Autodesk Inventor part; units mm, degrees
ref_plane "YZ Plane" through (0, 0, 0) normal (1, 0, 0) x (0, 1, 0)
ref_plane "XZ Plane" through (0, 0, 0) normal (0, 1, 0) x (-1, 0, 0)
ref_plane "XY Plane" through (0, 0, 0) normal (0, 0, 1) x (1, 0, 0)
sketch "Эскиз1" plane through (0, 0, 0) normal (0, 0, 1) x (1, 0, 0)
  line L0 (-69.2132, 0) -> (64.0355, 0)
  line L1 (0, -42.2487) -> (0, 42.2487)
  line L2 (-20, 25) -> (45, 25)
  line L3 (45, 25) -> (45, -25)
  line L4 (45, -25) -> (-20, -25)
  line L5 (-45, 0) -> (-45, 0)
  arc A0 (-20, 25) -> (-45, 0) centre (-20, 0) ccw
  arc A1 (-45, 0) -> (-20, -25) centre (-20, 0) ccw
  point P0 (0, 0)
  point P1 (-45, 25)
  dimension "d0" = 50
  dimension "d1" = 90
  dimension "d2" = 25
extrude "Выдавливание1" add sketch "Эскиз1" along normal blind 15
sketch "Эскиз2" plane through (0, 0, 15) normal (0, 0, 1) x (1, 0, 0)
  line L0 (45, -25) -> (45, 25)
  circle A0 centre (-10, 0) radius 14
  point P0 (0, 0)
  point P1 (30, 14.0013)
  point P2 (31.2898, -16.1928)
  dimension "d6" = 15
  dimension "d7" = 40
  dimension "d8" = 28
extrude "Выдавливание2" add sketch "Эскиз2" along normal blind 25
sketch "Эскиз3" plane through (-10, 0, 40) normal (0, 0, 1) x (1, 0, 0)
  point P0 (10, 0)
sketch "Эскиз4" plane through (-10, 0, 40) normal (0, 0, 1) x (1, 0, 0)
  point P0 (10, 0)
  point P1 (0, 0)
hole "Отверстие1" at (-10, 0, 40) direction (0, 0, -1) diameter 15.835 depth 30
chamfer "Фаска1" distance 2 angle 45 1 edges at (-10, 7.9175, 40)
sketch "Эскиз5" plane through (0, 0, 15) normal (0, 0, 1) x (1, 0, 0)
  line L0 (45, -25) -> (45, 25)
  circle A0 centre (-10, 0) radius 7.9175
  line L1 (-63, 0) -> (63, 0)
  line L2 (0, -35) -> (0, 35)
  point P0 (0, 0)
  point P1 (30, 15)
  point P2 (30, -15)
  dimension "d21" = 15
  dimension "d22" = 40
  dimension "d23" = 30
hole "Отверстие2" at (30, 15, 15) at (30, -15, 15) direction (0, 0, -1) diameter 10 end through all
properties part number "Основание дз курганова"
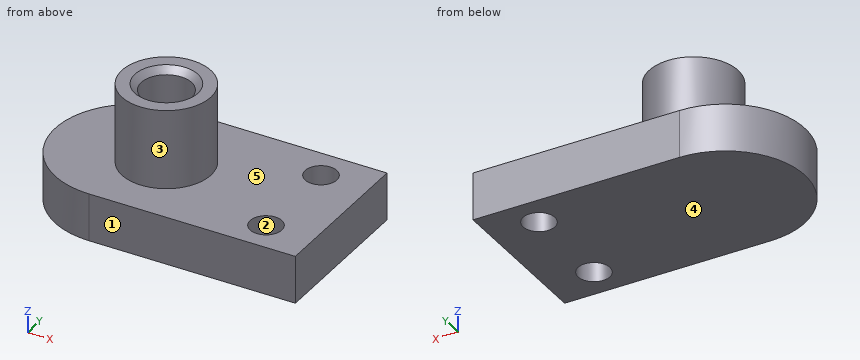
For this review, take the finished solid that the model builds, in its own axes (mm). Face numbers are marked on the shaded views. A direction names the side the tool comes from. Round coordinates to 2 decimals unless told otherwise and drop trailing zeros. Loops run counter-clockwise (first coordinate to the right, second up) from the corner with the lowest first, then second, coordinate; pieces in that order, holes last. Notation, with made-up numbers: (-16, 26.25) - (15, 26.25) arc R22 ccw to (15, 53.25) - close; hole circle Ø3 at (-26.5, 49). An arc over 180 degrees is marked (long way). One line per item, written item: value. Start each with the question number.
Item 1: The part is to be moulded in two halves that separate along X. For the marked faces 1, 2 and 3, say which applies: +X half, -X half, draft (parallel to the pull), parting line (faces both ways), or undercut.
Item 2: Take a section at A-A (y = 15). Give the boundary of the cut face in (x, z), plus the area to 4 significant figures.
Item 3: Clearance check with flat-ended pins moving along their axes: pin 1 Ø3 at (x, y) = (-31.5, -11.5) entering from +Z; pin 2 Ø10 at (y, z) = (-16, 15) entering from -X; pin 3 Ø10 at (y, z) = (-7, 29) entering from -X; pin 4 Ø9 at (x, y) = (30, 15) entering from +Z. State where each tip first meets the part, or that it passes through.
Item 4: Take a section at C-C (x = -10). Give the boundary of the cut face in (y, z).
Item 5: Take a section at B-B (x = 30). Give the boundary of the cut face in (y, z), plus the area to 3 significant figures.
Item 6: For L1, parallel to Y at x = 30, z = 4; L2, parallel to Y at x = -10, z = 16.5; L3, parallel to Z at x = 23, y = 8, list the stretches that pass through material, from the lowest coordinate up.
Item 7: Take a section at D-D (z = 26.5). Give the boundary of the cut face in (x, y) (1 decimal), plus the area to 3 significant figures.
Item 8: For the marked faces 4 and 5, list the 3-axis set-ups (+Z, -Z, +X, -X, +Y, -Y) from which the entire face can be reached by the end or side of a thin tool; tool diameter is ignored.
Answer below:
1. face 1: draft
1. face 2: undercut
1. face 3: parting line
2. outline: (-40, 0) - (25, 0) - (25, 15) - (-40, 15) - close; (35, 0) - (45, 0) - (45, 15) - (35, 15) - close
2. area: 1,125 mm2
3. pin 1: stops at z = 15
3. pin 2: stops at x = -42.45
3. pin 3: stops at x = -23.86
3. pin 4: passes through
4. outline: (-25, 0) - (25, 0) - (25, 15) - (14, 15) - (14, 40) - (9.92, 40) - (7.92, 38) - (7.92, 10) - (-7.92, 10) - (-7.92, 38) - (-9.92, 40) - (-14, 40) - (-14, 15) - (-25, 15) - close
5. outline: (-25, 0) - (-20, 0) - (-20, 15) - (-25, 15) - close; (-10, 0) - (10, 0) - (10, 15) - (-10, 15) - close; (20, 0) - (25, 0) - (25, 15) - (20, 15) - close
5. area: 450 mm2
6. L1: y = -25 to -20, -10 to 10, 20 to 25
6. L2: y = -14 to -7.92, 7.92 to 14
6. L3: z = 0 to 15
7. outline: circle Ø28 at (-10, 0); hole circle Ø15.8 at (-10, 0)
7. area: 419 mm2
8. face 4: -Z, +X, -X, +Y, -Y
8. face 5: +Z
